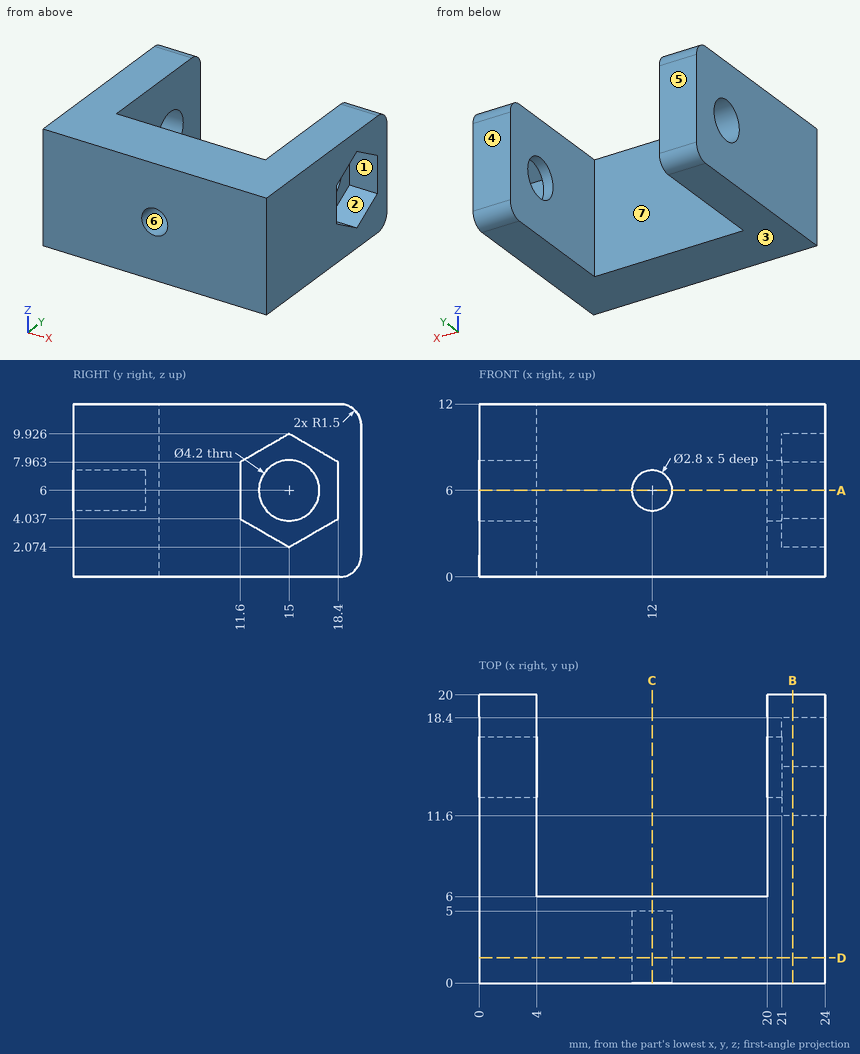
Geometry check sheet. Reference: drawing and pictorial views, mm from the part's lowest x, y, z. A direction names the side the tool comes from. Coordinates: 2 decimals unless noted, no trailing zeros. Order: outer loops, then holes, each group sorted by start corner. A loop starts at its lowest first (then second) coordinate and runs counter-clockwise, first axis right, second up.
Item 1: Section check D-D, the plane y = 1.75. Enter the section's corners in (x, z).
Filled in:
outline: (0, 0) - (24, 0) - (24, 12) - (0, 12) - close; hole circle Ø2.8 at (12, 6)
Item 2: Material ranges on L1, parallel to X at y = 7.75, z = 7.5; L2, parallel to X at y = 12.75, z = 4; L3, parallel to Z at x = 1.85, y = 15, recorded low to high.
Filled in:
L1: x = 0 to 4, 20 to 24
L2: x = 0 to 4, 20 to 21
L3: z = 0 to 3.9, 8.1 to 12
Item 3: Section check C-C, the plane x = 12. Enter the section's corners in (y, z).
Filled in:
outline: (0, 0) - (6, 0) - (6, 12) - (0, 12) - (0, 7.4) - (5, 7.4) - (5, 4.6) - (0, 4.6) - close
Item 4: Section check B-B, the plane x = 21.75. Enter the section's corners in (y, z).
Filled in:
outline: (0, 0) - (18.5, 0) arc R1.5 ccw to (20, 1.5) - (20, 10.5) arc R1.5 ccw to (18.5, 12) - (0, 12) - close; hole (11.6, 4.04) - (15, 2.07) - (18.4, 4.04) - (18.4, 7.96) - (15, 9.93) - (11.6, 7.96) - close
Item 5: Release check for a two-part mould opening along Z. For the marked faces 1, 2, 3 and 4 record: +Z half, -Z half, draft (parallel to the pull), parting line (faces both ways), or undercut.
Filled in:
face 1: undercut
face 2: undercut
face 3: -Z half
face 4: draft
Item 6: Access from +Z, -Z, +X, -X, +Y, -Y to the whole of each face (thin tool, end or side, straight path). Record for the marked faces 5, 6 and 7.
Filled in:
face 5: +Z, -Z, +X, -X, +Y
face 6: -Y
face 7: +Z, -Z, +Y
Item 7: Depth check by flat-ended pin: pin 1 (2 mm diameter, centred on x = 7, z = 8, fed in from -Y); pin 2 (3 mm diameter, centred on y = 14.5, z = 6, fed in from -X); pin 3 (3.5 mm diameter, centred on x = 10, z = 7, fed in from +Y); pin 4 (5.5 mm diameter, centred on y = 15, z = 6, fed in from +X). Enter the tip coordinate at first touch or a pass-through.
Filled in:
pin 1: stops at y = 0
pin 2: passes through
pin 3: stops at y = 6
pin 4: stops at x = 21
Item 8: Section check A-A, the plane z = 6. Enter the section's corners in (x, y), then the cut area to 3 significant figures.
Filled in:
outline: (0, 0) - (10.6, 0) - (10.6, 5) - (13.4, 5) - (13.4, 0) - (24, 0) - (24, 11.6) - (21, 11.6) - (21, 12.9) - (20, 12.9) - (20, 6) - (4, 6) - (4, 12.9) - (0, 12.9) - close; (0, 17.1) - (4, 17.1) - (4, 20) - (0, 20) - close; (20, 17.1) - (21, 17.1) - (21, 18.4) - (24, 18.4) - (24, 20) - (20, 20) - close
area: 201 mm2
